Could you check a few things on this drawing? It's one solid part, dimensions in mm from its lowest x, y, z. Coordinates: 2 decimals unless noted, no trailing zeros. Write each loop counter-clockwise with the first axis right and the second up, starting at its lowest first coordinate (ties: lowest second). Pieces come first, ordered by that corner, then holes.
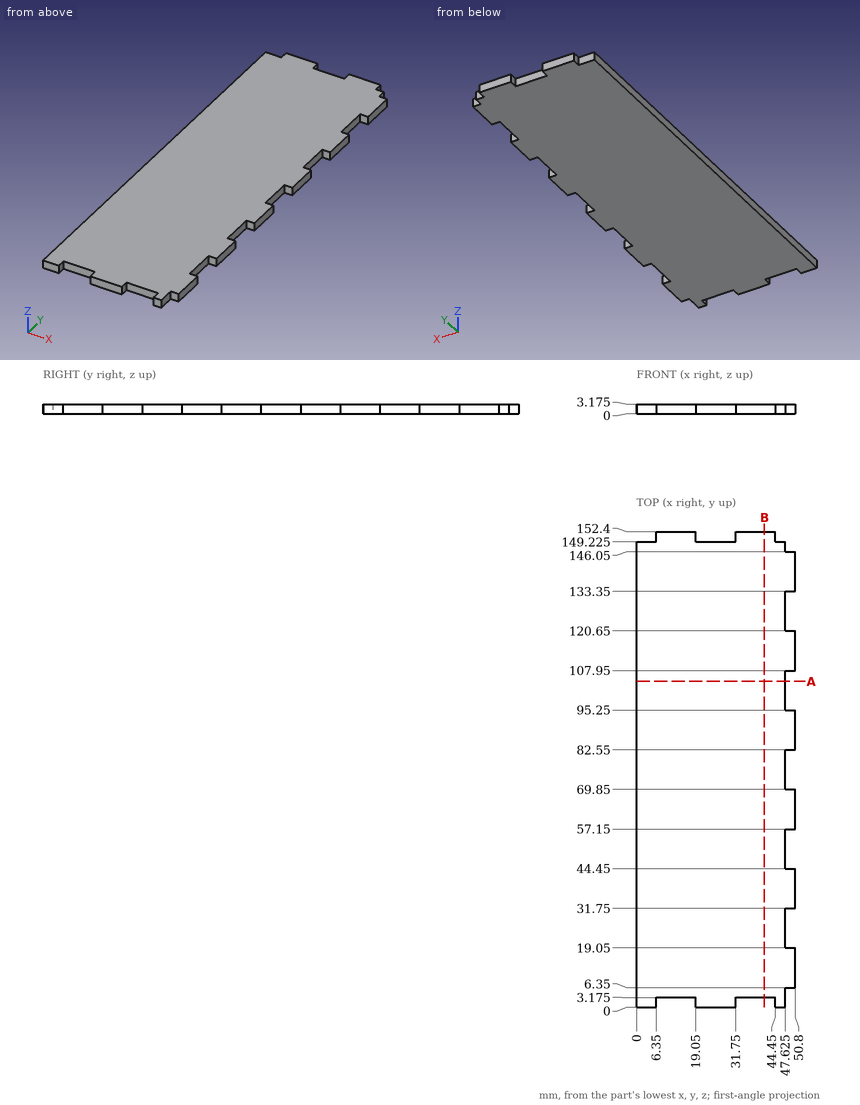
1) Imagine slicing it at A-A on y = 104.5. Please give me the cut outline in (x, z) (3 decimals), then the cut area to 3 significant figures.
Values follow:
outline: (0, 0) - (47.625, 0) - (47.625, 3.175) - (0, 3.175) - close
area: 151 mm2
2) Will these pins go through, and if not, where does the flat tip stop? pin 1 (4 mm diameter, centred on x = 37, y = 123, fed in from -Z); pin 2 (1 mm diameter, centred on y = 24, z = 1, fed in from +X) (3 decimals); pin 3 (1.6 mm diameter, centred on y = 151, z = 1, fed in from +X); pin 4 (1.6 mm diameter, centred on x = 24.5, z = 2, fed in from +Y) (3 decimals).
Values follow:
pin 1: stops at z = 0
pin 2: stops at x = 47.625
pin 3: stops at x = 44.45
pin 4: stops at y = 149.225
3) Imagine slicing it at B-B on x = 41. Please give me the cut outline in (y, z) (3 decimals), then the cut area to 3 significant figures.
Values follow:
outline: (3.175, 0) - (152.4, 0) - (152.4, 3.175) - (3.175, 3.175) - close
area: 474 mm2
4) I need wall thicknesses on probe 1 along Y at (x, z) = (44, 1.6) (3 decimals); probe 2 along X at (y, z) = (56, 2.8) (3 decimals); probe 3 along Y at (x, z) = (47, 0.9) (3 decimals). Which ranges of each line are inside material? Lowest first, please.
Values follow:
probe 1: y = 3.175 to 152.4
probe 2: x = 0 to 47.625
probe 3: y = 0 to 149.225
